from build123d import *

# Parameters (mm, degrees)
SKETCH1_W           = 92.0242
SKETCH1_H           = 61.4426
BOSS_EXTRUDE1_DEPTH = 8.89
SKETCH2_W           = 86.9442
SKETCH2_H           = 56.3626
CUT_EXTRUDE4_DEPTH  = 6.35
SKETCH3_W           = 5.08
SKETCH3_H           = 5.08
BOSS_EXTRUDE2_DEPTH = 8.7884
CUT_EXTRUDE5_DEPTH  = 5.08


with BuildPart() as part:
    # Sketch1 → Boss-Extrude1 (new body)
    with BuildSketch(Plane(origin=(0, 0, 0), x_dir=(1, 0, 0), z_dir=(0, 1, 0))):
        Rectangle(SKETCH1_W, SKETCH1_H)
    extrude(amount=-BOSS_EXTRUDE1_DEPTH)

    # Sketch2 → Cut-Extrude4 (cut)
    with BuildSketch(Plane(origin=(0, 0, 0), x_dir=(1, 0, 0), z_dir=(0, 1, 0))):
        Rectangle(SKETCH2_W, SKETCH2_H)
    extrude(amount=-CUT_EXTRUDE4_DEPTH, mode=Mode.SUBTRACT)

    # Sketch3 → Boss-Extrude2 (add)
    with BuildSketch(Plane.XZ.offset(8.89)):
        with Locations((37.7571, -22.4663)):
            Rectangle(SKETCH3_W, SKETCH3_H)
        with Locations((-37.7571, 22.4663)):
            Rectangle(SKETCH3_W, SKETCH3_H)
        with Locations((-37.7571, -22.4663)):
            Rectangle(SKETCH3_W, SKETCH3_H)
        with Locations((37.7571, 22.4663)):
            Rectangle(SKETCH3_W, SKETCH3_H)
    extrude(amount=BOSS_EXTRUDE2_DEPTH)

    # Sketch4 → Cut-Extrude5 (cut)
    with BuildSketch(Plane.XY.offset(25.0063)):
        Polygon((35.2171, -13.876876095), (35.2171, -17.6784), (37.7571, -17.6784), align=None)
        Polygon((35.2171, -8.89), (35.2171, -12.606876095), (36.938174553, -12.068216701), (36.938174553, -8.89), align=None)
        Polygon((-37.7571, -17.6784), (-40.2971, -13.876876095), (-40.2971, -17.6784), align=None)
        Polygon((-38.576025447, -12.068216701), (-38.576025447, -8.89), (-40.2971, -8.89), (-40.2971, -12.606876095), align=None)
    cut_extrude5 = extrude(amount=-CUT_EXTRUDE5_DEPTH, mode=Mode.SUBTRACT)

    # Mirror1: Cut-Extrude5 across plane
    add(cut_extrude5.mirror(Plane.XY), mode=Mode.SUBTRACT)


solid = part.part
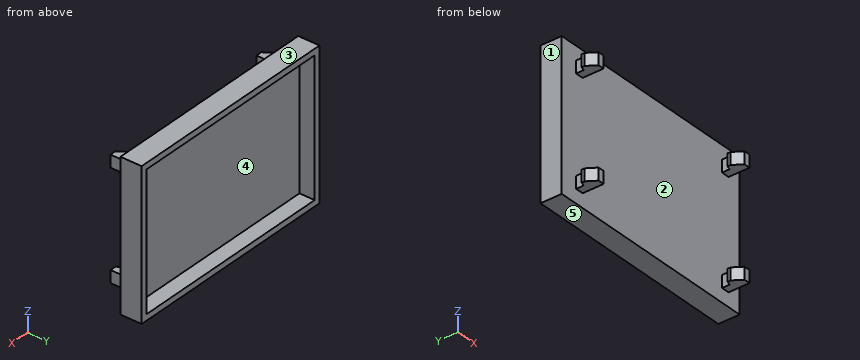
The listing builds one solid part. Answer for the finished solid, in the listing's coordinates (mm). Face numbers are marked on the shaded views. A direction names the side the tool comes from. Give positions to 0.01 mm unless a question says otherwise; leave off trailing zeros. Write each loop counter-clockwise with the first axis right and the second up, starting at its lowest first coordinate (ties: lowest second). Pieces come first, ordered by that corner, then holes. Notation, with made-up numbers: (65, 45) -> (115, 45) arc R33 cw to (115, 73) -> close; hole circle Ø1 at (42.5, 89). An arc over 180 degrees is marked (long way). One line per question, with ' | ' between items. Start each with the question number.
1. For the marked faces 4 and 5, determine the directions among +Z, -Z, +X, -X, +Y, -Y from which every point of the face is accessible in a straight line to the end or side of a thin tool.
2. Find the intervals of material crossed by probe 1 along X at (y, z) = (-4, -4.5); probe 2 along Z at (x, y) = (-35, -2); probe 3 along Y at (x, z) = (-3, 23.5), in increasing order.
3. Section B-B (z = 1) is taken. Determine the outline of the cut face in (x, y), plus the area to 3 significant figures.
4. Section D-D (x = 9.5) is taken. Determine the outline of the cut face in (y, z).
5. Given pin 1 Ø1.4 at (y, z) = (-13, 23.5) entering from -X; pin 2 Ø2.5 at (x, y) = (38, -11.5) entering from +Z; pin 3 Ø2 at (x, z) = (24, -12.5) entering from -Y, each flat-ended and moving along its own axis, determine where each tip first touches the part or whether it passes through.
6. For a pull along X with two mould halves and no side action, classify the marked faces 1, 2 and 3 as pulls with the +X half, pulls with the -X half, needs draft (parallel to the pull), parting line crosses it, or undercut.
7. Section A-A (y = -1.75) is taken. Determine the outline of the cut face in (x, z), plus the area to 3 significant figures.
8. Section C-C (y = -15.75) is taken. Determine the outline of the cut face in (x, z), plus the area to 3 significant figures.
Response values:
1) face 4: +Y | face 5: -Z, +X, -X, +Y, -Y
2) probe 1: -46.01 to -43.47, 43.47 to 46.01 | probe 2: -30.72 to -28.18, 28.18 to 30.72 | probe 3: -8.89 to -6.35
3) outline: (-46.01, -8.89) -> (46.01, -8.89) -> (46.01, 0) -> (43.47, 0) -> (43.47, -6.35) -> (-43.47, -6.35) -> (-43.47, 0) -> (-46.01, 0) -> close | area: 266 mm2
4) outline: (-8.89, -30.72) -> (0, -30.72) -> (0, -28.18) -> (-6.35, -28.18) -> (-6.35, 28.18) -> (0, 28.18) -> (0, 30.72) -> (-8.89, 30.72) -> close
5) pin 1: x = -40.3 | pin 2: z = 25.01 | pin 3: y = -8.89
6) face 1: pulls with the -X half | face 2: undercut | face 3: needs draft
7) outline: (-46.01, -30.72) -> (46.01, -30.72) -> (46.01, 30.72) -> (-46.01, 30.72) -> close; hole (-43.47, -28.18) -> (43.47, -28.18) -> (43.47, 28.18) -> (-43.47, 28.18) -> close | area: 754 mm2
8) outline: (-39.05, -25.01) -> (-35.22, -25.01) -> (-35.22, -19.93) -> (-39.05, -19.93) -> close; (-39.05, 19.93) -> (-35.22, 19.93) -> (-35.22, 25.01) -> (-39.05, 25.01) -> close; (36.47, -25.01) -> (40.3, -25.01) -> (40.3, -19.93) -> (36.47, -19.93) -> close; (36.47, 19.93) -> (40.3, 19.93) -> (40.3, 25.01) -> (36.47, 25.01) -> close | area: 77.8 mm2
